```python
from build123d import *

# Parameters (mm, degrees)
CROQUIS1_W              = 22
CROQUIS1_H              = 47
SALIENTE_EXTRUIR1_DEPTH = 3
CROQUIS2_W              = 22
CROQUIS2_H              = 3
SALIENTE_EXTRUIR2_DEPTH = 30
SALIENTE_EXTRUIR3_DEPTH = 11
CROQUIS5_R              = 2
CORTAR_EXTRUIR1_DEPTH   = 45.969434064


with BuildPart() as part:
    # Croquis1 → Saliente-Extruir1 (new body)
    with BuildSketch(Plane(origin=(0, 0, 0), x_dir=(1, 0, 0), z_dir=(0, 1, 0))):
        Rectangle(CROQUIS1_W, CROQUIS1_H)
    extrude(amount=SALIENTE_EXTRUIR1_DEPTH)

    # Croquis2 → Saliente-Extruir2 (add)
    with BuildSketch(Plane.XZ):
        with Locations((0, 22)):
            Rectangle(CROQUIS2_W, CROQUIS2_H)
        with Locations((0, -22)):
            Rectangle(CROQUIS2_W, CROQUIS2_H)
    extrude(amount=SALIENTE_EXTRUIR2_DEPTH)

    # Croquis4 → Saliente-Extruir3 (add, symmetric)
    with BuildSketch(Plane(origin=(0, 0, 0), x_dir=(0, 0, -1), z_dir=(1, 0, 0))):
        Polygon((23.5, -30), (28.5, -30), (28.5, -22), (23.5, -17), align=None)
    saliente_extruir3 = extrude(amount=SALIENTE_EXTRUIR3_DEPTH, both=True)

    # Croquis5 → Cortar-Extruir1 (cut, symmetric)
    with BuildSketch(Plane.XZ.offset(30)):
        with Locations(Location((5, -24.5, 0), (0, 0, 150))):
            Circle(CROQUIS5_R)
        with Locations(Location((-5, -24.5, 0), (0, 0, 150))):
            Circle(CROQUIS5_R)
    cortar_extruir1 = extrude(amount=CORTAR_EXTRUIR1_DEPTH, both=True, mode=Mode.SUBTRACT)

    # Simetría1: Saliente-Extruir3, Cortar-Extruir1 across plane
    add(saliente_extruir3.mirror(Plane.XY))
    add(cortar_extruir1.mirror(Plane.XY), mode=Mode.SUBTRACT)


solid = part.part
```
Design review of the part built by this model. Coordinates are the model's own, in mm. A direction names the side the tool comes from. Give positions to 0.01 mm unless a question says otherwise; leave off trailing zeros. Order: outer loops, then holes, each group sorted by start corner. A loop starts at its lowest first (then second) coordinate and runs counter-clockwise, first axis right, second up. Notation, with made-up numbers: (68.5, 22) - (75.5, 22) arc R24 ccw to (75.5, 38) - close; hole circle Ø1 at (-33, -14). An arc over 180 degrees is marked (long way). Use a Markdown table: item, result. Add a question column.
(1) Add section C-C on x = 5. Give the boundary of the cut face in (y, z).
(2) Wall thickness on probe 1 along Z at (x, y) = (5, -28.5); probe 2 along X at (y, z) = (-18.5, -24.5); probe 3 along Z at (x, y) = (5, -17.5): over which ranges is each line inside the solid? List them lowest first. Write a range as [from, to].
(3) Add section B-B on y = -2.5. Give the boundary of the cut face in (x, z), then the cut area to 3 significant figures.
(4) Add section A-A on y = -25. Give the boundary of the cut face in (x, z).
(5) Add section D-D on z = 24.5. Give the boundary of the cut face in (x, y), then the cut area to 3 significant figures.
(6) Clearance check with flat-ended pins moving along their axes: P1, Ø3.5, axis at x = 9, y = -10, coming from the -Z side; P2, Ø1.5, axis at x = -3.5, z = 2, coming from the -Y side; P3, Ø5, axis at x = -0.5, y = -3.5, coming from the +Z side; P4, Ø3.5, axis at x = 5, z = 24.5, coming from the -Y side. State where each tip first meets the part, or that it passes through.
(7) Mouldability with a two-part tool opening along Z and no side actions: class faces 1 (the face through (0, -26, 28.5)), 2 (the face through (-9, -7, -23.5)), 3 (the face through (-4.912, -17.398, 22.502)) as +Z half, -Z half, draft (parallel to the pull), parting line (faces both ways), or undercut.
(8) Machinability: for faces 4 (the face through (0, -15, 20.5)), 5 (the face through (0, -7, 23.5)), 6 (the face through (5.088, -17.398, 22.502)), which of the approach directions +Z, -Z, +X, -X, +Y, -Y give a long, thin tool a straight path to every point of the face, cutting with its end or side? Answer none if there is none.
Report:
| question | item | result |
|---|---|---|
| 1 | outline | (-30, -28.5) - (-22, -28.5) - (-20, -26.5) - (-30, -26.5) - close; (-30, -22.5) - (3, -22.5) - (3, 22.5) - (-30, 22.5) - (-30, 20.5) - (0, 20.5) - (0, -20.5) - (-30, -20.5) - close; (-30, 26.5) - (-20, 26.5) - (-22, 28.5) - (-30, 28.5) - close |
| 2 | probe 1 | z = [-28.5, -26.5], [-22.5, -20.5], [20.5, 22.5], [26.5, 28.5] |
| 2 | probe 2 | x = [-11, -7], [-3, 3], [7, 11] |
| 2 | probe 3 | z = [-22.5, -20.5], [20.5, 22.5] |
| 3 | outline | (-11, -23.5) - (-6.73, -23.5) arc R2 cw to (-3.27, -23.5) - (3.27, -23.5) arc R2 cw to (6.73, -23.5) - (11, -23.5) - (11, -20.5) - (-11, -20.5) - close; (-11, 20.5) - (11, 20.5) - (11, 23.5) - (6.73, 23.5) arc R2 cw to (3.27, 23.5) - (-3.27, 23.5) arc R2 cw to (-6.73, 23.5) - (-11, 23.5) - close |
| 3 | area | 122 mm² |
| 4 | outline | (-11, -28.5) - (11, -28.5) - (11, -20.5) - (-11, -20.5) - close; (-11, 20.5) - (11, 20.5) - (11, 28.5) - (-11, 28.5) - close; hole circle Ø4 at (-5, -24.5); hole circle Ø4 at (-5, 24.5); hole circle Ø4 at (5, -24.5); hole circle Ø4 at (5, 24.5) |
| 5 | outline | (-11, -30) - (-7, -30) - (-7, -18) - (-11, -18) - close; (-3, -30) - (3, -30) - (3, -18) - (-3, -18) - close; (7, -30) - (11, -30) - (11, -18) - (7, -18) - close |
| 5 | area | 168 mm² |
| 6 | P1 | stops at z = -23.5 |
| 6 | P2 | stops at y = 0 |
| 6 | P3 | stops at z = 23.5 |
| 6 | P4 | passes through |
| 7 | face 1 | +Z half |
| 7 | face 2 | -Z half |
| 7 | face 3 | undercut |
| 8 | face 4 | +X, -X, -Y |
| 8 | face 5 | +Z, +X, -X, +Y |
| 8 | face 6 | +Y, -Y |
